Geometry: see drawing. Coordinates: mm, zero at the bounding-box minimum. A direction names the side the tool comes from. Give positions to 0.01 mm unless a question says otherwise; leave off trailing zeros. Write each loop counter-clockwise with the first axis right and the second up, starting at its lowest first coordinate (ties: lowest second). Pieces come first, ordered by that corner, then holes. Notation, with made-up numbers: (43.25, 51.5) - (71.25, 51.5) arc R13 cw to (71.25, 55.5) - close; hole circle Ø6 at (35.25, 84). An arc over 180 degrees is marked (long way). Use a Markdown table: item, result. Add a question column.
1. Section query D-D, the plane x = 62. Return loops of the section in (y, z).
2. Set-up query: the marked faces 1 and 2. Return all of +Z, -Z, +X, -X, +Y, -Y with unobstructed straight access to the full face (end or side cutting, diameter ignored); none if empty.
3. Section query C-C, the plane y = 20.25. Count the separate pieces of the cut face and the enclosed holes in it, plus the area to 3 significant figures.
4. Section query A-A, the plane z = 46.1. Return loops of the section in (x, y), plus the area to 3 significant figures.
5. Material intervals for probe 1 along X at (y, z) = (24.15, 46.1); probe 2 along Y at (x, z) = (19.5, 38.5); probe 3 along Z at (x, y) = (78, 15.75), sorted ascending.
6. Mould query, pull axis Z, two halves, no side actions, for the marked faces 3, 4, 5 and 6. Classes: released by +Z, released by -Z, zero draft, split by the parting line, or undercut.
7. Pin query (flat end, axial travel): pin 1 (6 mm diameter, centred on y = 20.5, z = 30.5, fed in from +X); pin 2 (3 mm diameter, centred on x = 12.5, y = 17, fed in from +Z); pin 3 (1.5 mm diameter, centred on y = 18, z = 29, fed in from -X). Return the tip coordinate at first contact, or that it passes through.
8. Section query B-B, the plane x = 48. Return loops of the section in (y, z).
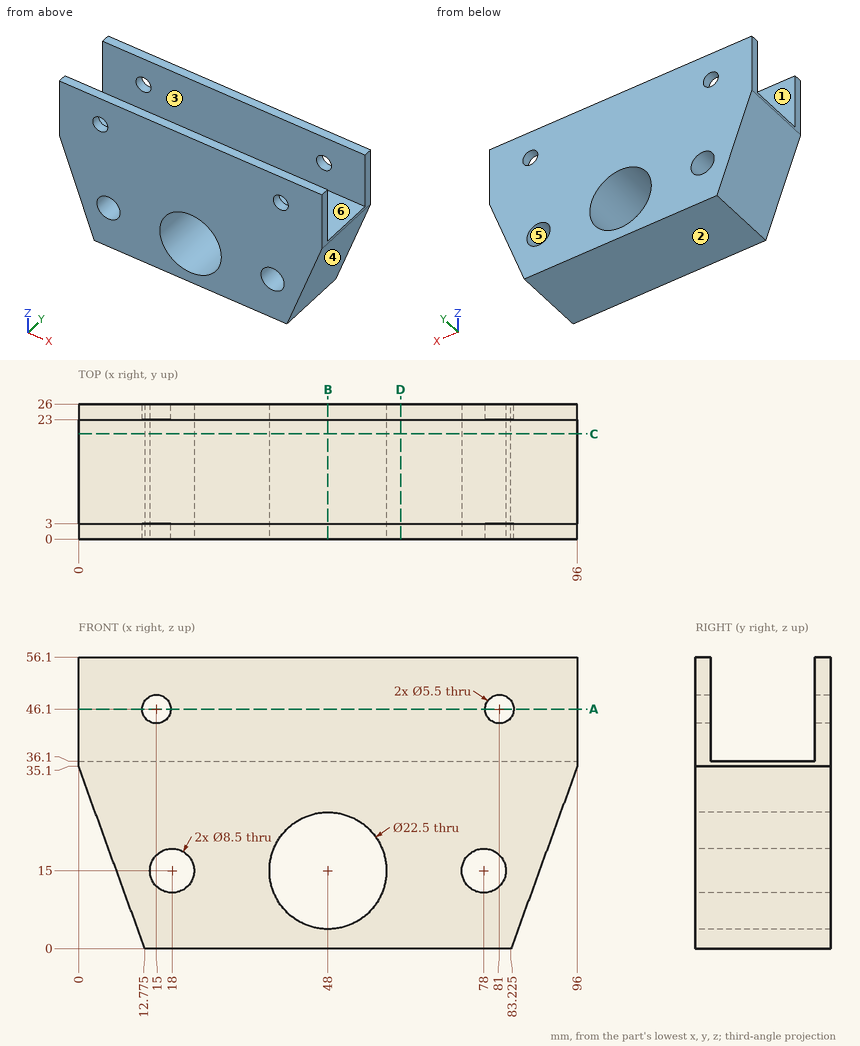
Result sheet:
| question | item | result |
|---|---|---|
| 1 | outline | (0, 0) - (26, 0) - (26, 56.1) - (23, 56.1) - (23, 36.1) - (3, 36.1) - (3, 56.1) - (0, 56.1) - close |
| 2 | face 1 | +Z, +X, -X |
| 2 | face 2 | -Z, +X, -X, +Y, -Y |
| 3 | separate pieces | 1 |
| 3 | enclosed holes | 3 |
| 3 | area | 2,510 mm² |
| 4 | outline | (0, 0) - (12.25, 0) - (12.25, 3) - (0, 3) - close; (0, 23) - (12.25, 23) - (12.25, 26) - (0, 26) - close; (17.75, 0) - (78.25, 0) - (78.25, 3) - (17.75, 3) - close; (17.75, 23) - (78.25, 23) - (78.25, 26) - (17.75, 26) - close; (83.75, 0) - (96, 0) - (96, 3) - (83.75, 3) - close; (83.75, 23) - (96, 23) - (96, 26) - (83.75, 26) - close |
| 4 | area | 510 mm² |
| 5 | probe 1 | x = 0 to 12.25, 17.75 to 78.25, 83.75 to 96 |
| 5 | probe 2 | y = 0 to 3, 23 to 26 |
| 5 | probe 3 | z = 0 to 10.75, 19.25 to 36.1 |
| 6 | face 3 | zero draft |
| 6 | face 4 | released by -Z |
| 6 | face 5 | undercut |
| 6 | face 6 | released by +Z |
| 7 | pin 1 | stops at x = 95.42 |
| 7 | pin 2 | stops at z = 36.1 |
| 7 | pin 3 | stops at x = 1.95 |
| 8 | outline | (0, 0) - (26, 0) - (26, 3.75) - (0, 3.75) - close; (0, 26.25) - (26, 26.25) - (26, 56.1) - (23, 56.1) - (23, 36.1) - (3, 36.1) - (3, 56.1) - (0, 56.1) - close |
